```python
from build123d import *

# Parameters (mm, degrees)
SKETCH1_R           = 5
SKETCH1_R_2         = 5.003763765
SKETCH1_R_3         = 4.999224106
SKETCH1_R_4         = 4
SKETCH1_R_5         = 2.510575716
SKETCH1_R_6         = 2.5
SKETCH1_R_7         = 3
SKETCH1_R_8         = 3.000476209
BOSS_EXTRUDE2_DEPTH = 5
SKETCH2_R           = 15
CUT_EXTRUDE1_DEPTH  = 7
SKETCH3_R           = 23.5
SKETCH3_R_2         = 21
BOSS_EXTRUDE4_DEPTH = 7
SKETCH4_R           = 30.235
SKETCH4_R_2         = 23.5
BOSS_EXTRUDE5_DEPTH = 18


with BuildPart() as part:
    # Sketch1 → Boss-Extrude2 (new body)
    # profile 1 of 4: a face of its own
    with BuildSketch(Plane(origin=(0, 0, 0), x_dir=(1, 0, 0), z_dir=(0, 1, 0))):
        with BuildLine():
            ThreePointArc((98.745189573, 22.608483412), (135.745189573, -14.391516588), (98.745189573, -51.391516588))
            Line((98.745189573, -51.391516588), (42.750189573, -51.391516588))
            ThreePointArc((42.750189573, -51.391516588), (6.260402135, -60.813200818), (-25.419810427, -40.401516588))
            Line((-25.419810427, -40.401516588), (-72.919810427, -40.401516588))
            Line((-72.919810427, -40.401516588), (-72.919810427, 11.578483412))
            Line((-72.919810427, 11.578483412), (-25.419810427, 11.578483412))
            ThreePointArc((-25.419810427, 11.578483412), (6.249075219, 32.009532595), (42.745189573, 22.608483412))
            Line((42.745189573, 22.608483412), (98.745189573, 22.608483412))
        make_face()
        with Locations(Location((34.750094787, -35.73, 0), (0, 0, 270))):
            Circle(SKETCH1_R, mode=Mode.SUBTRACT)
        with Locations(Location((-7.249905213, -35.74, 0), (0, 0, 270))):
            Circle(SKETCH1_R_2, mode=Mode.SUBTRACT)
        with Locations(Location((34.750094787, 6.25, 0), (0, 0, 270))):
            Circle(SKETCH1_R_3, mode=Mode.SUBTRACT)
        with Locations(Location((-7.25, 6.25, 0), (0, 0, 270))):
            Circle(SKETCH1_R, mode=Mode.SUBTRACT)
        with Locations(Location((-8.259097292, -14.412316007, 0), (0, 0, 270))):
            Circle(SKETCH1_R_4, mode=Mode.SUBTRACT)
        with Locations(Location((58.780189573, 15.578483412, 0), (0, 0, 270))):
            Circle(SKETCH1_R_5, mode=Mode.SUBTRACT)
        with Locations(Location((58.780189573, -44.401516588, 0), (0, 0, 270))):
            Circle(SKETCH1_R_6, mode=Mode.SUBTRACT)
        with Locations(Location((22.750189573, -53.411516588, 0), (0, 0, 270))):
            Circle(SKETCH1_R_6, mode=Mode.SUBTRACT)
        with Locations(Location((4.750189573, -53.411516588, 0), (0, 0, 270))):
            Circle(SKETCH1_R_6, mode=Mode.SUBTRACT)
        with Locations(Location((22.750189573, 24.588483412, 0), (0, 0, 270))):
            Circle(SKETCH1_R_6, mode=Mode.SUBTRACT)
        with Locations(Location((4.750189573, 24.588483412, 0), (0, 0, 270))):
            Circle(SKETCH1_R_6, mode=Mode.SUBTRACT)
        with Locations(Location((-43.249810427, 3.588483412, 0), (0, 0, 270))):
            Circle(SKETCH1_R_6, mode=Mode.SUBTRACT)
        with Locations(Location((-43.249810427, -32.411516588, 0), (0, 0, 270))):
            Circle(SKETCH1_R_6, mode=Mode.SUBTRACT)
        with Locations(Location((-64.219810427, -25.408584333, 0), (0, 0, 270))):
            Circle(SKETCH1_R_6, mode=Mode.SUBTRACT)
        with Locations(Location((-64.25, -3.408584333, 0), (0, 0, 270))):
            Circle(SKETCH1_R_6, mode=Mode.SUBTRACT)
    # profile 2 of 4: a face of its own
    with BuildSketch(Plane(origin=(0, 0, 0), x_dir=(1, 0, 0), z_dir=(0, 1, 0))):
        with BuildLine():
            Line((98.745189573, -51.391516588), (90.745189573, -51.391516588))
            Line((90.745189573, -51.391516588), (90.745189573, -56.389870622))
            ThreePointArc((90.745189573, -56.389870622), (94.745189573, -60.389870622), (98.745189573, -56.389870622))
            Line((98.745189573, -56.389870622), (98.745189573, -51.391516588))
        make_face()
        with Locations(Location((94.745189573, -56.389870622, 0), (0, 0, 270))):
            Circle(SKETCH1_R_7, mode=Mode.SUBTRACT)
    # profile 3 of 4: a face of its own
    with BuildSketch(Plane(origin=(0, 0, 0), x_dir=(1, 0, 0), z_dir=(0, 1, 0))):
        with BuildLine():
            ThreePointArc((135.528803249, -10.395798263), (135.745189573, -14.391516588), (135.528803249, -18.387234913))
            Line((135.528803249, -18.387234913), (139.748478132, -18.387234913))
            ThreePointArc((139.748478132, -18.387234913), (143.744196457, -14.391516588), (139.748478132, -10.395798263))
            Line((139.748478132, -10.395798263), (135.528803249, -10.395798263))
        make_face()
        with Locations(Location((139.748478132, -14.391516588, 0), (0, 0, 270))):
            Circle(SKETCH1_R_8, mode=Mode.SUBTRACT)
    # profile 4 of 4: a face of its own
    with BuildSketch(Plane(origin=(0, 0, 0), x_dir=(1, 0, 0), z_dir=(0, 1, 0))):
        with BuildLine():
            Line((90.745189573, 27.608483412), (90.745189573, 22.608483412))
            Line((90.745189573, 22.608483412), (98.745189573, 22.608483412))
            Line((98.745189573, 22.608483412), (98.745189573, 27.608483412))
            ThreePointArc((98.745189573, 27.608483412), (94.745189573, 31.608483412), (90.745189573, 27.608483412))
        make_face()
        with Locations(Location((94.745189573, 27.608483412, 0), (0, 0, 270))):
            Circle(SKETCH1_R_7, mode=Mode.SUBTRACT)
    extrude(amount=BOSS_EXTRUDE2_DEPTH)

    # Sketch2 → Cut-Extrude1 (cut)
    with BuildSketch(Plane(origin=(0, 5, 0), x_dir=(1, 0, 0), z_dir=(0, 1, 0))):
        with Locations(Location((98.745189573, -14.391516588, 0), (0, 0, 270))):
            Circle(SKETCH2_R)
    extrude(amount=-CUT_EXTRUDE1_DEPTH, mode=Mode.SUBTRACT)

    # Sketch3 → Boss-Extrude4 (add)
    with BuildSketch(Plane(origin=(0, 5, 0), x_dir=(1, 0, 0), z_dir=(0, 1, 0))):
        with Locations(Location((98.745189573, -14.391516588, 0), (0, 0, 270))):
            Circle(SKETCH3_R)
        with Locations(Location((98.745189573, -14.391516588, 0), (0, 0, 270))):
            Circle(SKETCH3_R_2, mode=Mode.SUBTRACT)
    extrude(amount=BOSS_EXTRUDE4_DEPTH)

    # Sketch4 → Boss-Extrude5 (add)
    with BuildSketch(Plane(origin=(0, 5, 0), x_dir=(1, 0, 0), z_dir=(0, 1, 0))):
        with Locations(Location((98.745189573, -14.391516588, 0), (0, 0, 270))):
            Circle(SKETCH4_R)
        with Locations(Location((98.745189573, -14.391516588, 0), (0, 0, 270))):
            Circle(SKETCH4_R_2, mode=Mode.SUBTRACT)
    extrude(amount=BOSS_EXTRUDE5_DEPTH)


solid = part.part
```
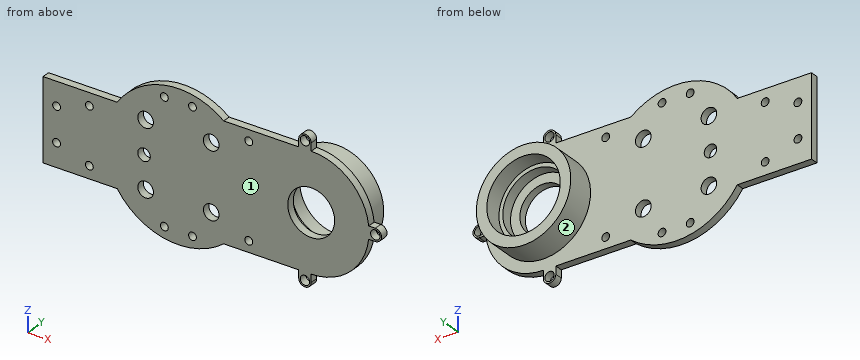
Read the model definition and answer for the solid it produces. Units are mm, in the model's axes. Face numbers are marked on the shaded views. A direction names the side the tool comes from. Give positions to 0.01 mm unless a question says otherwise; leave off trailing zeros. Write each loop counter-clockwise with the first axis right and the second up, starting at its lowest first coordinate (ties: lowest second). Pieces come first, ordered by that corner, then holes. Notation, with made-up numbers: M 36.5,51.5 L 82.5,51.5 A11 cw 82.5,56.5 Z; hole C -30.75,22 d1. An arc over 180 degrees is marked long. Put each result on its own line as item: value. Start each with the question number.
1. The part is cut by section A-A, the plane y = 9. Give the vertices of the cut face in (x, z) (3 decimals), and give its area (3 significant figures).
2. Each of these flat-tipped pins is pushed along its axis until it touches: pin 1 Ø2.5 at (y, z) = (2, -26) entering from +X; pin 2 Ø10 at (y, z) = (6.5, 4) entering from +X; pin 3 Ø3 at (x, z) = (12, 48) entering from +Y. Where does it stop, or does it pass through?
3. Consider line 1 along X through (y, z) = (4.5, 39); line 2 along X through (y, z) = (2.5, -5); line 3 along Y through (x, z) = (-54.5, 16.5). Determine where each line is inside the solid, lowest interval first.
4. The part is cut by section B-B, the plane x = -56. Give the vertices of the cut face in (y, z).
5. Which of the six approach directions +Z, -Z, +X, -X, +Y, -Y give full straight-line access (tool end or side, diameter ignored) to the marked faces 1 and 2?
Final values:
1. outline: C 98.745,14.392 d60.47; hole C 98.745,14.392 d42
1. area: 1,490 mm²
2. pin 1: stops at x = 98.75
2. pin 2: stops at x = 135.32
2. pin 3: stops at y = 5
3. line 1: x = -72.92 to -11.05, -3.45 to 30.97, 38.53 to 126.38
3. line 2: x = -72.92 to -45.31, -41.19 to -12.09, -2.41 to 29.91, 39.59 to 130.26
3. line 3: y = 0 to 5
4. outline: M 0,-11.58 L 5,-11.58 L 5,40.4 L 0,40.4 Z
5. face 1: +Z, -Z, +X, -X, -Y
5. face 2: +Y
